The model under review builds one solid part; all positions refer to its coordinate system, in mm. A direction names the side the tool comes from. Coordinates: 2 decimals unless noted, no trailing zeros. Write each loop counter-clockwise with the first axis right and the second up, starting at its lowest first coordinate (ties: lowest second). Pieces come first, ordered by that corner, then holes. Notation, with made-up numbers: (0, -34.75) - (45, -34.75) arc R15 cw to (45, -23.75) - close; hole circle Ø10 at (30, -18.75). An arc over 180 degrees is marked (long way). Return JSON: item names as keys, results as strings. Group by question number.
(1) Tool access review of faces 1 (the face through (-19, 0, 10)), 2 (the face through (0, 1, 21)): name each direction out of +Z, -Z, +X, -X, +Y, -Y from which nothing blocks a thin tool from reaching the whole face with its end or side.
(2) We need section B-B on z = 0. State the section outline as (x, y) points.
(3) We need section C-C on y = 0.7. State the section outline as (x, z) points.
(4) Draft analysis for pull direction Z (two halves, no side actions). For faces 3 (the face through (14, 1, 17.324)), 4 (the face through (10, 0.2, 23)), 5 (the face through (7.36, 1.58, 23.37)), state which applies: released by +Z, released by -Z, zero draft, split by the parting line, or undercut.
(5) We need section A-A on x = 0. State the section outline as (y, z) points, then the cut area to 3 significant figures.
(6) For pin 1 Ø1 at (y, z) = (2.5, -14) entering from -X; pin 2 Ø1.5 at (x, y) = (-13.5, 1) entering from -Z; pin 3 Ø1.5 at (x, y) = (-13, 1.5) entering from +Z, all flat-tipped, find the tip position at first contact; note any pin that passes through.
(7) To check wall thickness, follow L1, parallel to X at y = 0.3, z = -11; L2, parallel to Z at x = -17, y = 1.25; L3, parallel to X at y = 0.5, z = -1. State the ranges of each line that lie inside material, in increasing order. Write a range as from..to.
```python
from build123d import *

# Parameters (mm, degrees)
SKETCH_1_R          = 24.5
SKETCH_1_R_2        = 21
EXTRUDE_1_DEPTH     = 3
SKETCH_2_R          = 25.5
SKETCH_2_R_2        = 24.5
EXTRUDE_2_DEPTH     = 0.2
CUT_EXTRUDE_START   = -3
CUT_EXTRUDE_3_DEPTH = 3


with BuildPart() as part:
    # 草图1 → 凸台-拉伸1 (new body)
    with BuildSketch(Plane(origin=(0, 0, 0), x_dir=(1, 0, 0), z_dir=(0, 1, 0))):
        with Locations(Location((0, 0, 0), (0, 0, 270))):
            Circle(SKETCH_1_R)
        with Locations(Location((0, 0, 0), (0, 0, 270))):
            Circle(SKETCH_1_R_2, mode=Mode.SUBTRACT)
    extrude(amount=EXTRUDE_1_DEPTH)

    # 草图2 → 凸台-拉伸2 (add)
    with BuildSketch(Plane.XZ):
        with Locations(Location((0, 0, 0), (0, 0, 270))):
            Circle(SKETCH_2_R)
        with Locations(Location((0, 0, 0), (0, 0, 270))):
            Circle(SKETCH_2_R_2, mode=Mode.SUBTRACT)
    extrude(amount=-EXTRUDE_2_DEPTH)

    # 草图3 → 切除-拉伸3 (cut)
    with BuildSketch(Plane(origin=(0, 3, 0), x_dir=(1, 0, 0), z_dir=(0, 1, 0)).offset(CUT_EXTRUDE_START)):
        with BuildLine():
            Line((-15.324116139, 17.324116139), (15.324116139, 17.324116139))
            ThreePointArc((15.324116139, 17.324116139), (16.738329701, 16.738329701), (17.324116139, 15.324116139))
            Line((17.324116139, 15.324116139), (17.324116139, -15.324116139))
            ThreePointArc((17.324116139, -15.324116139), (16.738329701, -16.738329701), (15.324116139, -17.324116139))
            Line((15.324116139, -17.324116139), (-15.324116139, -17.324116139))
            ThreePointArc((-15.324116139, -17.324116139), (-16.738329701, -16.738329701), (-17.324116139, -15.324116139))
            Line((-17.324116139, -15.324116139), (-17.324116139, 15.324116139))
            ThreePointArc((-17.324116139, 15.324116139), (-16.738329701, 16.738329701), (-15.324116139, 17.324116139))
        make_face()
    extrude(amount=CUT_EXTRUDE_3_DEPTH, mode=Mode.SUBTRACT)


solid = part.part
```
Ans:
{
 "1": {"face 1": "+Z, -Z, +X, -X, -Y", "face 2": "+Y, -Y"},
 "2": {"outline": "(-25.5, 0) - (-21, 0) - (-21, 3) - (-24.5, 3) - (-24.5, 0.2) - (-25.5, 0.2) - close; (21, 0) - (25.5, 0) - (25.5, 0.2) - (24.5, 0.2) - (24.5, 3) - (21, 3) - close"},
 "3": {"outline": "circle Ø49 at (0, 0); hole (-17.32, -15.32) arc R2 ccw to (-15.32, -17.32) - (-11.87, -17.32) arc R21 ccw to (11.87, -17.32) - (15.32, -17.32) arc R2 ccw to (17.32, -15.32) - (17.32, -11.87) arc R21 ccw to (17.32, 11.87) - (17.32, 15.32) arc R2 ccw to (15.32, 17.32) - (11.87, 17.32) arc R21 ccw to (-11.87, 17.32) - (-15.32, 17.32) arc R2 ccw to (-17.32, 15.32) - (-17.32, 11.87) arc R21 ccw to (-17.32, -11.87) - close"},
 "4": {"face 3": "undercut", "face 4": "zero draft", "face 5": "split by the parting line"},
 "5": {"outline": "(0, -25.5) - (0.2, -25.5) - (0.2, -24.5) - (3, -24.5) - (3, -21) - (0, -21) - close; (0, 21) - (3, 21) - (3, 24.5) - (0.2, 24.5) - (0.2, 25.5) - (0, 25.5) - close", "area": "21.4 mm²"},
 "6": {"pin 1": "x = -20.45", "pin 2": "z = -20.92", "pin 3": "z = 21.22"},
 "7": {"L1": "-21.89..-17.89, 17.89..21.89", "L2": "-17.64..-16.42, 16.42..17.64", "L3": "-24.48..-20.98, 20.98..24.48"}
}
